Verification items for the finished model (mm, model axes). A direction names the side the tool comes from. Give positions to 0.01 mm unless a question says otherwise; leave off trailing zeros. Loops run counter-clockwise (first coordinate to the right, second up) from the corner with the lowest first, then second, coordinate; pieces in that order, holes last. Notation, with made-up numbers: (3, -34) - (21, -34) arc R18 ccw to (21, -2) - close; hole circle Ø9 at (-37.75, -29.5). An arc over 180 degrees is marked (long way). One line per question, with ' | ' between items. Start each with the question number.
1. Mould release check, pull along Z, two halves, no side actions. Record for faces 5 (the face through (77.457, -31.665, 46.881)), 6 (the face through (-8, 201.66, 33)): +Z half, -Z half, draft (parallel to the pull), parting line (faces both ways), or undercut.
2. Depth check by flat-ended pin: pin 1 Ø1.5 at (x, z) = (25, 29) entering from -Y; pin 2 Ø6.5 at (y, z) = (181.66, 33.5) entering from -X; pin 3 Ø20 at (x, z) = (36, 41) entering from +Y; pin 4 Ø10 at (x, y) = (-4, 135) entering from -Z. Enter the tip coordinate at first touch or a pass-through.
3. Section check A-A, the plane z = 33.5. Enter the section's corners in (x, y).
4. Thickness scan on line 1 along X through (y, z) = (69, 10.5); line 2 along Y through (x, z) = (63.5, 20.5); line 3 along Y through (x, z) = (-3, 33). Record the ranges inside material, lowest first. Write a range as from..to.
5. Section check C-C, the plane y = 57.5. Enter the section's corners in (x, z).
6. Section check D-D, the plane z = 62.5. Enter the section's corners in (x, y).
7. Tool access check on faces 1 (the face through (68.331, 155, 33)), 2 (the face through (-7.543, -26.842, 22.632)), 3 (the face through (35, 23.66, 33)), 4 (the face through (68.331, 66, 33)). Record the directions out of +Z, -Z, +X, -X, +Y, -Y that give a thin tool (end or side, any length) a straight path to the whole face; none if there is none.
8. Section check B-B, the plane x = 63.5. Enter the section's corners in (y, z), then the cut area to 3 significant figures.
from build123d import *

# Parameters (mm, degrees)
SKETCH1_W           = 67
SKETCH1_H           = 50
BOSS_EXTRUDE3_DEPTH = 67
SKETCH2_R           = 3
SKETCH2_R_2         = 4
CUT_EXTRUDE1_DEPTH  = 18
CUT_EXTRUDE2_START  = -18
SKETCH3_R           = 3
SKETCH3_R_2         = 4
CUT_EXTRUDE2_DEPTH  = 18


with BuildPart() as part:
    # Sketch1 → Boss-Extrude3 (new body)
    with BuildSketch(Plane.XY):
        Polygon((1.330634734, 23.660498279), (1.330634734, -98.339501721), (-16.669365266, -98.339501721), (-16.669365266, 201.660498279), (1.330634734, 201.660498279), (1.330634734, 109.660498279), (68.330634734, 109.660498279), (68.330634734, 201.660498279), (86.330634734, 201.660498279), (86.330634734, -98.339501721), (68.330634734, -98.339501721), (68.330634734, 23.660498279), align=None)
        with Locations((34.830634734, 66.660498279)):
            Rectangle(SKETCH1_W, SKETCH1_H, mode=Mode.SUBTRACT)
    extrude(amount=BOSS_EXTRUDE3_DEPTH)

    # Sketch2 → Cut-Extrude1 (cut)
    with BuildSketch(Plane(origin=(86.330634734, 0, 0), x_dir=(0, 0, -1), z_dir=(1, 0, 0))):
        with Locations((-44.5, -29.839501721)):
            Circle(SKETCH2_R)
        with Locations((-22.5, -7.339501721)):
            Circle(SKETCH2_R)
        with Locations((-33.5, 181.660498279)):
            Circle(SKETCH2_R_2)
    extrude(amount=-CUT_EXTRUDE1_DEPTH, mode=Mode.SUBTRACT)

    # Sketch3 → Cut-Extrude2 (cut)
    with BuildSketch(Plane.ZY.offset(16.669365266).offset(CUT_EXTRUDE2_START)):
        with Locations(Location((22.5, -29.839501721, 0), (0, 0, 270))):
            Circle(SKETCH3_R)
        with Locations(Location((44.5, -7.339501721, 0), (0, 0, 270))):
            Circle(SKETCH3_R)
        with Locations(Location((33.5, 181.660498279, 0), (0, 0, 180))):
            Circle(SKETCH3_R_2)
    extrude(amount=CUT_EXTRUDE2_DEPTH, mode=Mode.SUBTRACT)


solid = part.part
Results list:
1) face 5: undercut | face 6: draft
2) pin 1: y = 23.66 | pin 2: through | pin 3: y = 109.66 | pin 4: z = 0
3) outline: (-16.67, -98.34) - (1.33, -98.34) - (1.33, 23.66) - (68.33, 23.66) - (68.33, -98.34) - (86.33, -98.34) - (86.33, 177.66) - (68.33, 177.66) - (68.33, 109.66) - (1.33, 109.66) - (1.33, 177.66) - (-16.67, 177.66) - close; (-16.67, 185.66) - (1.33, 185.66) - (1.33, 201.66) - (-16.67, 201.66) - close; (68.33, 185.66) - (86.33, 185.66) - (86.33, 201.66) - (68.33, 201.66) - close; hole (1.33, 41.66) - (68.33, 41.66) - (68.33, 91.66) - (1.33, 91.66) - close
4) line 1: -16.67..1.33, 68.33..86.33 | line 2: 23.66..41.66, 91.66..109.66 | line 3: -98.34..177.69, 185.63..201.66
5) outline: (-16.67, 0) - (1.33, 0) - (1.33, 67) - (-16.67, 67) - close; (68.33, 0) - (86.33, 0) - (86.33, 67) - (68.33, 67) - close
6) outline: (-16.67, -98.34) - (1.33, -98.34) - (1.33, 23.66) - (68.33, 23.66) - (68.33, -98.34) - (86.33, -98.34) - (86.33, 201.66) - (68.33, 201.66) - (68.33, 109.66) - (1.33, 109.66) - (1.33, 201.66) - (-16.67, 201.66) - close; hole (1.33, 41.66) - (68.33, 41.66) - (68.33, 91.66) - (1.33, 91.66) - close
7) face 1: +Z, -Z, +Y | face 2: -X | face 3: +Z, -Z, -Y | face 4: +Z, -Z
8) outline: (23.66, 0) - (41.66, 0) - (41.66, 67) - (23.66, 67) - close; (91.66, 0) - (109.66, 0) - (109.66, 67) - (91.66, 67) - close | area: 2,410 mm²
